Here's the drawing with two shaded views (mm, measured from the low corner). I have some questions. A direction names the side the tool comes from. Coordinates: 2 decimals unless noted, no trailing zeros. Write each loop counter-clockwise with the first axis right and the second up, starting at its lowest first coordinate (ties: lowest second). Pieces come first, ordered by that corner, then holes. Notation, with made-up numbers: (70.25, 60.5) -> (100.25, 60.5) arc R24 ccw to (100.25, 71.5) -> close; hole circle Ø3 at (28.5, 89.25). An arc over 180 degrees is marked (long way). Use one line per item in the form item = value.
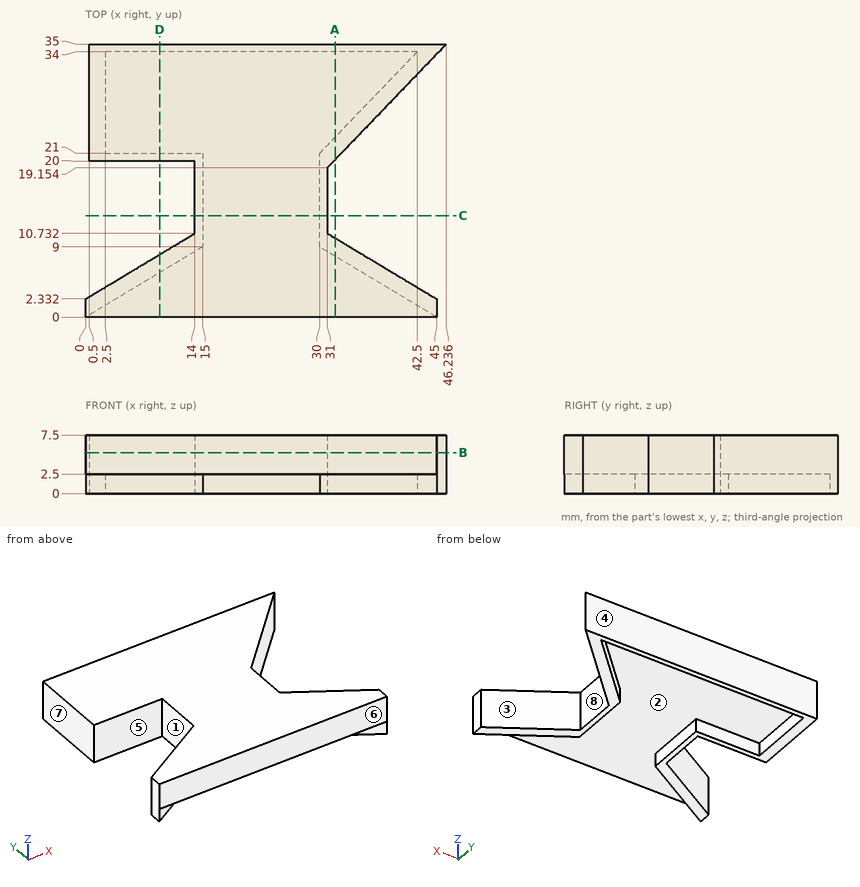
Q1. For the marked faces 5, 6, 7 and 8, which set-ups out of +Z, -Z, +X, -X, +Y, -Y let a thin tool reach every point of the face, with its end or its side?
Return value:
face_5 = +Z, -Z, -X
face_6 = +Z, -Z, +X, -X, -Y
face_7 = +Z, -Z, -X, +Y
face_8 = +Z, -Z, +X
Q2. If I drill on line 1 (X direction, y = 12, z = 1.25); line 2 (Y direction, x = 38, z = 2.25) (1 decimal); line 3 (Z direction, x = 33, y = 7), over which ranges is the centre line in solid material (lowest first)? Write a range as from..to.
Return value:
line_1 = 14..15, 30..31
line_2 = 4.2..6.5, 26.4..29.3, 34..35
line_3 = 2.5..7.5
Q3. Suppose I cut it at D-D (x = 9.5). Write out the boundary of the cut face in (y, z), then the cut area to 3 significant figures.
Return value:
outline = (0, 2.5) -> (5.7, 2.5) -> (5.7, 0) -> (8.03, 0) -> (8.03, 7.5) -> (0, 7.5) -> close; (20, 0) -> (21, 0) -> (21, 2.5) -> (34, 2.5) -> (34, 0) -> (35, 0) -> (35, 7.5) -> (20, 7.5) -> close
area = 126 mm2
Q4. Suppose I cut it at B-B (z = 5.25). Write out the boundary of the cut face in (x, y) (1 decimal), then the cut area to 3 significant figures.
Return value:
outline = (0, 0) -> (45, 0) -> (45, 2.3) -> (31, 10.7) -> (31, 19.2) -> (46.2, 35) -> (0.5, 35) -> (0.5, 20) -> (14, 20) -> (14, 10.7) -> (0, 2.3) -> close
area = 1,100 mm2
Q5. Will these pins go through, and if not, where does the flat tip stop? pin 1 (2 mm diameter, centred on y = 24, z = 2, fed in from -X); pin 2 (3 mm diameter, centred on y = 12.5, z = 1, fed in from -X); pin 3 (1 mm diameter, centred on x = 29, y = 27.5, fed in from -Z).
Return value:
pin_1 = 0.5
pin_2 = 14
pin_3 = 2.5
Q6. Thinking about a two-plate mould opening in X: for the marked faces 1, 2, 3 and 4, which applies, released by +X, released by -X, zero draft, split by the parting line, or undercut?
Return value:
face_1 = released by -X
face_2 = undercut
face_3 = released by +X
face_4 = zero draft
Q7. Suppose I cut it at A-A (x = 32). Write out the boundary of the cut face in (y, z) (1 decimal), then the cut area to 3 significant figures.
Return value:
outline = (0, 2.5) -> (7.8, 2.5) -> (7.8, 0) -> (10.1, 0) -> (10.1, 7.5) -> (0, 7.5) -> close; (20.2, 0) -> (23.1, 0) -> (23.1, 2.5) -> (34, 2.5) -> (34, 0) -> (35, 0) -> (35, 7.5) -> (20.2, 7.5) -> close
area = 140 mm2
Q8. Suppose I cut it at C-C (y = 13). Write out the boundary of the cut face in (x, z).
Return value:
outline = (14, 0) -> (15, 0) -> (15, 2.5) -> (30, 2.5) -> (30, 0) -> (31, 0) -> (31, 7.5) -> (14, 7.5) -> close
